Verification items for the finished model (mm, model axes). A direction names the side the tool comes from. Round coordinates to 2 decimals unless told otherwise and drop trailing zeros. Write each loop counter-clockwise with the first axis right and the second up, starting at its lowest first coordinate (ties: lowest second). Pieces come first, ordered by that corner, then holes. Notation, with made-up numbers: M 60.5,-26 L 97.5,-26 A19 cw 97.5,-22 Z; hole C -13.75,-27 d9. An arc over 180 degrees is marked long. One line per question, with ' | ' between items.
from build123d import *

# Parameters (mm, degrees)
PAD_DEPTH    = 55
PAD001_DEPTH = 2
SKETCH001_R  = 1.5
POCKET_DEPTH = 179.264648


with BuildPart() as part:
    # Sketch → Pad (new body)
    with BuildSketch(Plane.XY):
        with BuildLine():
            Line((11.5, 0), (13.5, 2))
            Line((13.5, 2), (11.5, 33.5))
            ThreePointArc((11.5, 33.5), (8.93934, 34.56066), (10, 32))
            Line((10, 32), (12, 4))
            Line((12, 4), (10.5, 2.5))
            Line((1, 2.5), (10.5, 2.5))
            Line((0, 4), (1, 2.5))
            Line((0, 4), (0, 0))
            Line((0, 0), (11.5, 0))
        make_face()
    pad = extrude(amount=PAD_DEPTH)

    # Mirrored: Pad across Sketch V_Axis
    add(pad.mirror(Plane(origin=(0, 0, 0), x_dir=(0, 0, 1), z_dir=(1, 0, 0))))

    # Sketch002 → Pad001 (join)
    with BuildSketch(Plane.XY):
        Polygon((11.5, 33.5), (7.5, 33.5), (7.5, 7.5), (13.5, 2), align=None)
        Polygon((11.5, 0), (7, 6), (0, 6), (0, 0), align=None)
    pad001 = extrude(amount=-PAD001_DEPTH)

    # Mirrored001: Pad001 across Sketch002 V_Axis
    add(pad001.mirror(Plane(origin=(0, 0, 0), x_dir=(0, 0, 1), z_dir=(1, 0, 0))))

    # Sketch001 → Pocket (cut, through all)
    with BuildSketch(Plane.XZ):
        with Locations((6, 6)):
            Circle(SKETCH001_R)
        with Locations((6, 49)):
            Circle(SKETCH001_R)
    pocket = extrude(amount=-POCKET_DEPTH, mode=Mode.SUBTRACT)

    # Mirrored002: Pocket across Sketch001 V_Axis
    add(pocket.mirror(Plane(origin=(0, 0, 0), x_dir=(0, -1, 0), z_dir=(1, 0, 0))), mode=Mode.SUBTRACT)


solid = part.part
1. Thickness scan on line 1 (Z direction, x = 6, y = 2); line 2 (Y direction, x = 1.5, z = 45); line 3 (Z direction, x = -10, y = 10). Record the ranges inside material, lowest first.
Results:
line 1: z = -2 to 4.5, 7.5 to 47.5, 50.5 to 55 | line 2: y = 0 to 2.5 | line 3: z = -2 to 0
2. Mould release check, pull along Z, two halves, no side actions. Record for faces 5 (the face through (-4.8, 1.2, 5.1)), 6 (the face through (0.1, 4.3, 0)), 7 (the face through (-12, 2, 0)), 8 (the face through (6, 2.5, 27)): pulls with the +Z half, pulls with the -Z half, needs draft (parallel to the pull), parting line crosses it, or undercut.
Results:
face 5: undercut | face 6: pulls with the +Z half | face 7: pulls with the -Z half | face 8: needs draft
3. Section check A-A, the plane z = 49. Record the cut outline in (x, y), then the cut area to 3 significant figures.
Results:
outline: M -13.5,2 L -11.5,0 L -7.5,0 L -7.5,2.5 L -10.5,2.5 L -12,4 L -10,32 A1.5 ccw long -11.5,33.5 Z; M -4.5,0 L 4.5,0 L 4.5,2.5 L 1,2.5 L 0,4 L -1,2.5 L -4.5,2.5 Z; M 7.5,0 L 11.5,0 L 13.5,2 L 11.5,33.5 A1.5 ccw long 10,32 L 12,4 L 10.5,2.5 L 7.5,2.5 Z | area: 155 mm2
4. Go/stop test with flat-tipped pins: P1, Ø0.7, axis at x = 10, y = 34, coming from the -Z side; P2, Ø1.5, axis at x = 3, z = 46.5, coming from the +Y side; P3, Ø2, axis at x = -0.5, z = -1.5, coming from the +Y side. Record where each tip stops, or that it passes through.
Results:
P1: stops at z = 0 | P2: stops at y = 2.5 | P3: stops at y = 6
5. Tool access check on faces 1 (the face through (-5.675, 1.232, 47.536)), 2 (the face through (11, 18, 27)), 3 (the face through (9.28, 2.96, -0.99)), 4 (the face through (-7.5, 21, -1)). Record the directions out of +Z, -Z, +X, -X, +Y, -Y that give a thin tool (end or side, any length) a straight path to the whole face; none if there is none.
Results:
face 1: +Y, -Y | face 2: +Z | face 3: -Z | face 4: +Z, -Z, +Y
6. Section check B-B, the plane x = 6. Record the cut outline in (y, z).
Results:
outline: M 0,-2 L 6,-2 L 6,0 L 2.5,0 L 2.5,4.5 L 0,4.5 Z; M 0,7.5 L 2.5,7.5 L 2.5,47.5 L 0,47.5 Z; M 0,50.5 L 2.5,50.5 L 2.5,55 L 0,55 Z
7. Section check C-C, the plane y = 18.5. Record the cut outline in (x, z).
Results:
outline: M -12.45,-2 L -7.5,-2 L -7.5,0 L -10.96,0 L -10.96,55 L -12.45,55 Z; M 7.5,-2 L 12.45,-2 L 12.45,55 L 10.96,55 L 10.96,0 L 7.5,0 Z
8. Section check D-D, the plane z = 32. Record the cut outline in (x, y).
Results:
outline: M -13.5,2 L -11.5,0 L 11.5,0 L 13.5,2 L 11.5,33.5 A1.5 ccw long 10,32 L 12,4 L 10.5,2.5 L 1,2.5 L 0,4 L -1,2.5 L -10.5,2.5 L -12,4 L -10,32 A1.5 ccw long -11.5,33.5 Z
